Verification items for the finished model (mm, model axes). A direction names the side the tool comes from. Round coordinates to 2 decimals unless told otherwise and drop trailing zeros. Order: outer loops, then holes, each group sorted by start corner. A loop starts at its lowest first (then second) coordinate and runs counter-clockwise, first axis right, second up. Notation, with made-up numbers: M 84,68.5 L 109,68.5 A31 cw 109,95.5 Z; hole C 62,62 d6. An arc over 180 degrees is marked long. Return JSON: item names as keys, results as strings. Group by question number.
Autodesk Inventor part; units mm, degrees
ref_plane "YZ Plane" through (0, 0, 0) normal (1, 0, 0) x (0, 1, 0)
ref_plane "XZ Plane" through (0, 0, 0) normal (0, 1, 0) x (-1, 0, 0)
ref_plane "XY Plane" through (0, 0, 0) normal (0, 0, 1) x (1, 0, 0)
sketch "Sketch1" plane through (0, 0, 0) normal (0, 0, 1) x (1, 0, 0)
  line L0 (-5.7947, 5.8302) -> (7.2053, 5.8302)
  line L1 (7.2053, 5.8302) -> (7.2053, -7.1698)
  line L2 (7.2053, -7.1698) -> (-5.7947, -7.1698)
  line L3 (-5.7947, -7.1698) -> (-5.7947, 5.8302)
  arc A0 (-5.7947, -7.1698) -> (-1.7947, 5.8302) centre (-34.6583, 8.8267) ccw
  arc A1 (3.2053, 5.8302) -> (7.2053, -7.1698) centre (36.069, 8.8267) ccw
  point P0 (0, 0)
  dimension "d0" = 13
  dimension "d1" = 13
  dimension "d2" = 4
  dimension "d3" = 4
  dimension "d4" = 33
  dimension "d5" = 33
extrude "Extrusion1" add sketch "Sketch1" along normal blind 8.976 contours L0 A1 L2 A0
sketch "Sketch2" plane through (-5.7947, -7.1698, 0) normal (0, -1, 0) x (1, 0, 0)
  line L0 (9.1, 5.238) -> (3.7, 5.238)
  line L1 (3.7, 5.238) -> (3.7, 3.738)
  line L2 (3.7, 3.738) -> (9.1, 3.738)
  line L3 (9.1, 3.738) -> (9.1, 5.238)
  line L4 (0, 8.976) -> (13, 8.976)
  line L5 (13, 0) -> (13, 8.976)
  point P0 (5.7947, 0)
  dimension "d8" = 1.5
  dimension "d9" = 5.4
  dimension "d10" = 3.738
  dimension "d11" = 3.9
extrude "Extrusion2" cut sketch "Sketch2" against normal blind 2
sketch "Sketch3" plane through (-5.7947, -5.1698, 0) normal (0, -1, 0) x (1, 0, 0)
  line L0 (9.1, 3.738) -> (3.7, 3.738)
  line L1 (4, 5.238) -> (8.8, 5.238)
  line L2 (8.8, 5.238) -> (8.8, 3.738)
  line L3 (8.8, 3.738) -> (4, 3.738)
  line L4 (4, 3.738) -> (4, 5.238)
  line L5 (3.7, 5.238) -> (9.1, 5.238)
  line L6 (3.7, 3.738) -> (3.7, 5.238)
  line L7 (9.1, 5.238) -> (9.1, 3.738)
  point P0 (5.7947, 0)
  dimension "d14" = 0
  dimension "d15" = 0.3
  dimension "d16" = 0.3
extrude "Extrusion3" cut sketch "Sketch3" against normal blind 10 contours L0 L4 L1 L2
fillet "Fillet1" radius 1 8 edges at (3.2053, 5.8302, 4.488) (-3.1176, -0.8781, 8.976) (0.7053, 5.8302, 8.976) (-1.7947, 5.8302, 4.488) (0.7053, 5.8302, 0) (4.5283, -0.8781, 0) (-3.1176, -0.8781, 0) (4.5283, -0.8781, 8.976)
properties part number "SingleSliderCap"
1. Draft check along Z on faces 1 (the face through (1, -1, 5.238)), 2 (the face through (0.728, 5.545, 8.675)), 3 (the face through (4.69, -1.39, 4.44)). Enter one of: +Z half, -Z half, draft (parallel to the pull), parting line (faces both ways), or undercut.
2. Thickness scan on line 1 along Z through (x, y) = (0, 2); line 2 along X through (y, z) = (-0.5, 4.25); line 3 along X through (y, z) = (-1.25, 1.25). Record the ranges inside material, lowest first. Write a range as from..to.
3. Go/stop test with flat-tipped pins: pin 1 (1.7 mm diameter, centred on y = 2, z = 4.5, fed in from +X); pin 2 (0.5 mm diameter, centred on y = -6.5, z = 4, fed in from +X); pin 3 (1.5 mm diameter, centred on y = -0.5, z = 1.5, fed in from +X). Record where each tip stops, or that it passes through.
4. Cross-section at B-B (z = 2). Enter the section's corners in (x, y), plus the area to 3 significant figures.
5. Access from +Z, -Z, +X, -X, +Y, -Y to the whole of each face (thin tool, end or side, straight path). Record for faces 4 (the face through (-1.551, 5.584, 4.537)), 5 (the face through (-1.795, 0, 4)).
6. Cross-section at A-A (x = 0). Enter the section's corners in (y, z).
Computed:
{
 "1": {"face 1": "undercut", "face 2": "+Z half", "face 3": "draft"},
 "2": {"line 1": "z = 0..3.74, 5.24..8.98", "line 2": "x = -3..-1.79, 3.01..4.41", "line 3": "x = -3.23..4.65"},
 "3": {"pin 1": "stops at x = 3.97", "pin 2": "stops at x = 6.98", "pin 3": "stops at x = 4.65"},
 "4": {"outline": "M -5.79,-7.17 L 7.21,-7.17 A33 cw 3.3,4.95 A1 ccw 2.3,5.83 L -0.89,5.83 A1 ccw -1.89,4.95 A33 cw Z", "area": "104 mm²"},
 "5": {"face 4": "+Z, -Z, -X, +Y", "face 5": "-Y"},
 "6": {"outline": "M -7.17,0 L 4.83,0 A1 ccw 5.83,1 L 5.83,7.98 A1 ccw 4.83,8.98 L -7.17,8.98 L -7.17,5.24 L 4.83,5.24 L 4.83,3.74 L -7.17,3.74 Z"}
}
